from build123d import *

# Parameters (mm, degrees)
CUT_EXTRUDE1_DEPTH = 10
FILLET1_R          = 10
SKETCH5_R          = 2
CUT_EXTRUDE2_DEPTH = 10


with BuildPart() as part:
    # Sketch3 → Revolve1 (revolve)
    with BuildSketch(Plane(origin=(0, 0, 0), x_dir=(0, 0, -1), z_dir=(1, 0, 0)), mode=Mode.PRIVATE) as revolve1_sk:
        Polygon((0, 12), (6, 12), (6, 8), (16, 8), (16, 12), (22, 12), (22, 35), (17, 35), (17, 17), (0, 17), align=None)
    revolve(revolve1_sk.sketch.rotate(Axis((0, 0, 0), (0, 0, -1)), 90), axis=Axis((0, 0, 0), (0, 0, -1)))

    # Sketch4 → Cut-Extrude1 (cut)
    with BuildSketch(Plane.XY.offset(-17)):
        with BuildLine():
            ThreePointArc((35, 0), (32.335783638, 13.393920133), (24.748737342, 24.748737342))
            Line((24.748737342, 24.748737342), (24.748737342, -24.748737342))
            ThreePointArc((24.748737342, -24.748737342), (32.335783638, -13.393920133), (35, 0))
        make_face()
        with BuildLine():
            ThreePointArc((24.748737342, 24.748737342), (0, 35), (-24.748737342, 24.748737342))
            Line((-24.748737342, 24.748737342), (24.748737342, 24.748737342))
        make_face()
        with BuildLine():
            Line((-24.748737342, -24.748737342), (-24.748737342, 24.748737342))
            ThreePointArc((-24.748737342, 24.748737342), (-35, 0), (-24.748737342, -24.748737342))
        make_face()
        with BuildLine():
            Line((24.748737342, -24.748737342), (-24.748737342, -24.748737342))
            ThreePointArc((-24.748737342, -24.748737342), (0, -35), (24.748737342, -24.748737342))
        make_face()
    extrude(amount=-CUT_EXTRUDE1_DEPTH, mode=Mode.SUBTRACT)

    # Fillet1
    fillet1_edges = [part.edges().sort_by_distance(p)[0] for p in [
        (24.748737342, 24.748737342, -19.5),
        (24.748737342, -24.748737342, -19.5),
        (-24.748737342, 24.748737342, -19.5),
        (-24.748737342, -24.748737342, -19.5),
    ]]
    fillet(fillet1_edges, radius=FILLET1_R)

    # Sketch5 → Cut-Extrude2 (cut)
    with BuildSketch(Plane(origin=(0, 0, -22), x_dir=(-1, 0, 0), z_dir=(0, 0, -1))):
        with Locations((-17.5, 17.5)):
            Circle(SKETCH5_R)
        with Locations((17.5, 17.5)):
            Circle(SKETCH5_R)
        with Locations((17.5, -17.5)):
            Circle(SKETCH5_R)
        with Locations((-17.5, -17.5)):
            Circle(SKETCH5_R)
    extrude(amount=-CUT_EXTRUDE2_DEPTH, mode=Mode.SUBTRACT)


solid = part.part
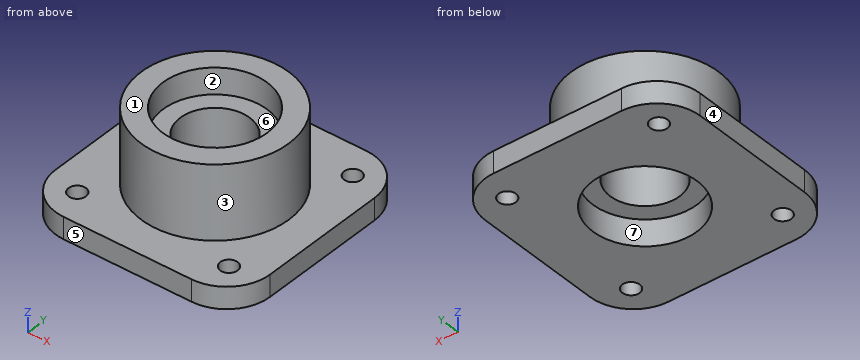
Input: part model. Units: mm. Frame: model coordinates. Face numbers are marked on the shaded views. A direction names the side the tool comes from. Coordinates: 2 decimals unless noted, no trailing zeros. Loops run counter-clockwise (first coordinate to the right, second up) from the corner with the lowest first, then second, coordinate; pieces in that order, holes last.
(1) Section C-C on z = -13.25. Return the cut outline in (x, y), then the cut area to 3 significant figures.
(2) Section D-D on x = -9. Return the cut outline in (y, z).
(3) First-contact query: pin 1 Ø7 at (x, y) = (2.5, 4) entering from +Z; pin 2 Ø6.5 at (x, y) = (17.5, 17.5) entering from +Z; pin 3 Ø1 at (y, z) = (6.5, -9) entering from -X; pin 4 Ø10 at (x, y) = (15.5, 7) entering from +Z. Flat tips, straight axial feed; report the tip coordinate or a pass-through.
(4) Set-up query: the marked faces 5, 6 and 7. Return all of +Z, -Z, +X, -X, +Y, -Y with unobstructed straight access to the full face (end or side cutting, diameter ignored); none if empty.
(5) Pull-direction query (X, two-part tool) for the marked faces 1, 2, 3 and 4; classes: released by +X, released by -X, zero draft, split by the parting line, or undercut.
(6) Section B-B on x = 5. Return the cut outline in (y, z) (3 decimals), then the cut area to 3 significant figures.
(7) Material intervals for probe 1 along Y at (x, z) = (17.5, -19.05); probe 2 along Y at (x, z) = (0, -1.2); probe 3 along Z at (x, y) = (9, -18.5), sorted ascending.
(8) Section A-A on y = 0. Return the cut outline in (x, z).
Data:
1. outline: circle Ø34 at (0, 0); hole circle Ø16 at (0, 0)
1. area: 707 mm2
2. outline: (-24.75, -22) - (-7.94, -22) - (-7.94, -16) - (7.94, -16) - (7.94, -22) - (24.75, -22) - (24.75, -17) - (14.42, -17) - (14.42, 0) - (7.94, 0) - (7.94, -6) - (-7.94, -6) - (-7.94, 0) - (-14.42, 0) - (-14.42, -17) - (-24.75, -17) - close
3. pin 1: stops at z = -6
3. pin 2: stops at z = -17
3. pin 3: stops at x = -15.91
3. pin 4: stops at z = 0
4. face 5: +Z, -Z, +X, -X, -Y
4. face 6: +Z
4. face 7: -Z
5. face 1: zero draft
5. face 2: undercut
5. face 3: split by the parting line
5. face 4: released by -X
6. outline: (-24.749, -22) - (-10.909, -22) - (-10.909, -16) - (-6.245, -16) - (-6.245, -6) - (-10.909, -6) - (-10.909, 0) - (-16.248, 0) - (-16.248, -17) - (-24.749, -17) - close; (6.245, -16) - (10.909, -16) - (10.909, -22) - (24.749, -22) - (24.749, -17) - (16.248, -17) - (16.248, 0) - (10.909, 0) - (10.909, -6) - (6.245, -6) - close
6. area: 413 mm2
7. probe 1: y = -24.36 to -19.5, -15.5 to 15.5, 19.5 to 24.36
7. probe 2: y = -17 to -12, 12 to 17
7. probe 3: z = -22 to -17
8. outline: (-24.75, -22) - (-12, -22) - (-12, -16) - (-8, -16) - (-8, -6) - (-12, -6) - (-12, 0) - (-17, 0) - (-17, -17) - (-24.75, -17) - close; (8, -16) - (12, -16) - (12, -22) - (24.75, -22) - (24.75, -17) - (17, -17) - (17, 0) - (12, 0) - (12, -6) - (8, -6) - close
